Input: part model. Units: mm. Frame: model coordinates. A direction names the side the tool comes from. Give positions to 0.01 mm unless a question says otherwise; leave off trailing zeros. Order: outer loops, then holes, each group sorted by start corner. A loop starts at its lowest first (then second) coordinate and runs counter-clockwise, first axis right, second up. Notation, with made-up numbers: (79.25, 78.25) - (129.25, 78.25) arc R12 ccw to (129.25, 84.25) - close; hole circle Ø3 at (-13.5, -2.75). An arc over 180 degrees is marked (long way). Answer in a Markdown table with one row per item. Add a question column.
1. Access query for faces 1 (the face through (-51, 1, -21)), 2 (the face through (-47, 1, -21)). Directions: +Z, -Z, +X, -X, +Y, -Y. A direction counts if a zero-diameter tool reaches every point of the face in a straight line with its end or side. Return the directions, or none.
2. Section query C-C on y = 1.45. Return loops of the section in (x, z).
3. Section query B-B on z = -5. Return loops of the section in (x, y).
4. Section query A-A on x = -24. Return loops of the section in (y, z), and give its area (3 significant figures).
5. Ray query, line 1 (Z direction, x = -41, y = 1.05); line 2 (X direction, y = 1.3, z = -5); line 3 (Z direction, x = -32, y = 0.75). Return the intervals inside material, ascending. Write a range as [from, to].
6. Mould query, pull axis Z, two halves, no side actions, for faces 3 (the face through (-26, 1, -42)), 4 (the face through (-25, 0, -35)), 5 (the face through (-25, 1, 0)), 6 (the face through (-26, 1, -29)). Classes: released by +Z, released by -Z, zero draft, split by the parting line, or undercut.
7. Section query D-D on z = -30.5. Return loops of the section in (x, y), and give its area (3 significant figures).
Autodesk Inventor part; units mm, degrees
ref_plane "YZ Plane" through (0, 0, 0) normal (1, 0, 0) x (0, 1, 0)
ref_plane "XZ Plane" through (0, 0, 0) normal (0, 1, 0) x (-1, 0, 0)
ref_plane "XY Plane" through (0, 0, 0) normal (0, 0, 1) x (1, 0, 0)
sketch "Sketch1" plane through (0, 0, 0) normal (0, 1, 0) x (-1, 0, 0)
  line L0 (0, 0) -> (51, 0)
  line L1 (51, 0) -> (51, -42)
  line L2 (51, -42) -> (0, -42)
  line L3 (0, -42) -> (0, 0)
  line L4 (51, -21) -> (0, -21)
  line L5 (25.5, 0) -> (25.5, -42)
  line L6 (41, -21) -> (10, -21) construction
  line L7 (41, -15) -> (10, -15)
  line L8 (10, -27) -> (41, -27)
  arc A0 (41, -27) -> (41, -15) centre (41, -21) ccw
  arc A1 (10, -15) -> (10, -27) centre (10, -21) ccw
  line L9 (41, -30.5) -> (10, -30.5) construction
  line L10 (41, -29) -> (10, -29)
  line L11 (10, -32) -> (41, -32)
  arc A2 (41, -32) -> (41, -29) centre (41, -30.5) ccw
  arc A3 (10, -29) -> (10, -32) centre (10, -30.5) ccw
  line L12 (41, -13) -> (10, -13)
  line L13 (10, -10) -> (41, -10)
  arc A4 (41, -13) -> (41, -10) centre (41, -11.5) ccw
  arc A5 (10, -10) -> (10, -13) centre (10, -11.5) ccw
  point P0 (41, -5)
  point P1 (41, -37)
  point P2 (10, -5)
  point P3 (10, -37)
  point P4 (25.5, -21)
  point P5 (35.9893, -30.5)
  point P6 (25.5, -30.5)
  point P7 (6, -5)
  point P8 (6, -37)
  dimension "d0" = 51
  dimension "d1" = 42
  dimension "d2" = 10
  dimension "d3" = 5
  dimension "d4" = 10
  dimension "d5" = 10
  dimension "d6" = 12
  dimension "d7" = 3.5
  dimension "d8" = 3
  dimension "d18" = 6
  dimension "d19" = 6
  dimension "d20" = 3.5
extrude "Extrusion1" add sketch "Sketch1" along normal blind 2 contours L0 L5 L13 A5 L12 L7 A1 L4 L3 | L0 L1 L4 A0 L7 L5 L12 A4 L13 | L4 A1 L8 L5 L10 A3 L11 L2 L3 | L1 L2 L5 L11 A2 L10 L8 A0 L4
hole "Hole1" at (-41, 0, -5) at (-41, 0, -37) at (-41, 0, -21) at (-10, 0, -21) at (-35.9893, 0, -30.5) at (-41, 0, -30.5) at (-10, 0, -30.5) at (-41, 0, -11.5) at (-10, 0, -11.5) at (-6, 0, -5) at (-6, 0, -37) direction (0, 1, 0) diameter 3 depth 43.75 tip angle 118
equation "\"d20\" = d7"
properties part number "temsion1" material "アルミニウム 6061"
Answer:
| question | item | result |
|---|---|---|
| 1 | face 1 | +Z, -Z, -X, +Y, -Y |
| 1 | face 2 | +Y, -Y |
| 2 | outline | (-51, -42) - (0, -42) - (0, 0) - (-51, 0) - close; hole circle Ø3 at (-41, -37); hole circle Ø3 at (-41, -5); hole (-41, -32) - (-10, -32) arc R1.5 ccw to (-10, -29) - (-41, -29) arc R1.5 ccw to start; hole (-41, -27) - (-10, -27) arc R6 ccw to (-10, -15) - (-41, -15) arc R6 ccw to start; hole (-41, -13) - (-10, -13) arc R1.5 ccw to (-10, -10) - (-41, -10) arc R1.5 ccw to start; hole circle Ø3 at (-6, -37); hole circle Ø3 at (-6, -5) |
| 3 | outline | (-51, 0) - (-42.5, 0) - (-42.5, 2) - (-51, 2) - close; (-39.5, 0) - (-7.5, 0) - (-7.5, 2) - (-39.5, 2) - close; (-4.5, 0) - (0, 0) - (0, 2) - (-4.5, 2) - close |
| 4 | outline | (0, -42) - (2, -42) - (2, -32) - (0, -32) - close; (0, -29) - (2, -29) - (2, -27) - (0, -27) - close; (0, -15) - (2, -15) - (2, -13) - (0, -13) - close; (0, -10) - (2, -10) - (2, 0) - (0, 0) - close |
| 4 | area | 48.0 mm² |
| 5 | line 1 | z = [-42, -38.5], [-35.5, -32], [-29, -27], [-15, -13], [-10, -6.5], [-3.5, 0] |
| 5 | line 2 | x = [-51, -42.5], [-39.5, -7.5], [-4.5, 0] |
| 5 | line 3 | z = [-42, -32], [-29, -27], [-15, -13], [-10, 0] |
| 6 | face 3 | released by -Z |
| 6 | face 4 | zero draft |
| 6 | face 5 | released by +Z |
| 6 | face 6 | undercut |
| 7 | outline | (-51, 0) - (-42.5, 0) - (-42.5, 2) - (-51, 2) - close; (-8.5, 0) - (0, 0) - (0, 2) - (-8.5, 2) - close |
| 7 | area | 34.0 mm² |
